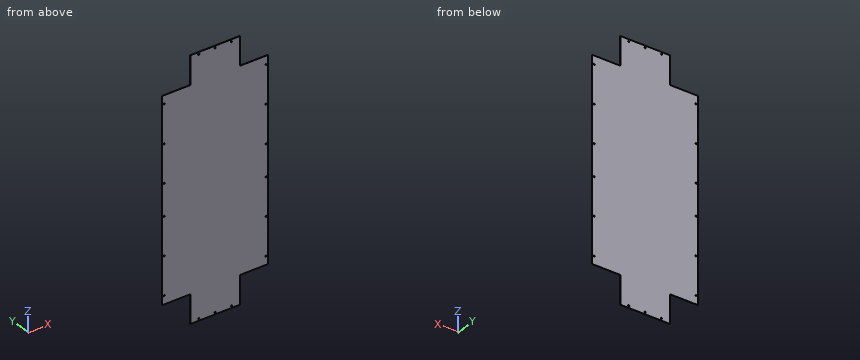
```python
from build123d import *

# Parameters (mm, degrees)
BASE_FLANGE1_DEPTH = 1
SKETCH6_R          = 3
CUT_EXTRUDE1_DEPTH = 10


# Sheet-metal steps are written as plain solids
with BuildPart() as part:
    # Sketch1 → Base-Flange1 (new body)
    with BuildSketch(Plane(origin=(0, 0, 0), x_dir=(1, 0, 0), z_dir=(0, 1, 0))):
        Polygon((135, 0), (371, 0), (371, 135), (506, 135), (506, 1085), (371, 1085), (371, 1220), (135, 1220), (135, 1085), (0, 1085), (0, 135), (135, 135), align=None)
    extrude(amount=-BASE_FLANGE1_DEPTH)

    # Sketch6 → Cut-Extrude1 (cut)
    with BuildSketch(Plane(origin=(0, 0, 0), x_dir=(1, 0, 0), z_dir=(0, 1, 0))):
        with Locations(Location((496, 1045, 0), (0, 0, 270))):
            Circle(SKETCH6_R)
        with Locations(Location((496, 865, 0), (0, 0, 270))):
            Circle(SKETCH6_R)
        with Locations(Location((496, 685, 0), (0, 0, 270))):
            Circle(SKETCH6_R)
        with Locations(Location((331, 1210, 0), (0, 0, 270))):
            Circle(SKETCH6_R)
        with Locations(Location((175, 1210, 0), (0, 0, 270))):
            Circle(SKETCH6_R)
        with Locations(Location((10, 685, 0), (0, 0, 270))):
            Circle(SKETCH6_R)
        with Locations(Location((10, 865, 0), (0, 0, 270))):
            Circle(SKETCH6_R)
        with Locations(Location((10, 1045, 0), (0, 0, 270))):
            Circle(SKETCH6_R)
        with Locations(Location((253, 1209.997298013, 0), (0, 0, 270))):
            Circle(SKETCH6_R)
        with Locations(Location((253, 10.002701987, 0), (0, 0, 270))):
            Circle(SKETCH6_R)
        with Locations(Location((10, 175, 0), (0, 0, 270))):
            Circle(SKETCH6_R)
        with Locations(Location((10, 355, 0), (0, 0, 270))):
            Circle(SKETCH6_R)
        with Locations(Location((10, 535, 0), (0, 0, 270))):
            Circle(SKETCH6_R)
        with Locations(Location((175, 10, 0), (0, 0, 270))):
            Circle(SKETCH6_R)
        with Locations(Location((331, 10, 0), (0, 0, 270))):
            Circle(SKETCH6_R)
        with Locations(Location((496, 535, 0), (0, 0, 270))):
            Circle(SKETCH6_R)
        with Locations(Location((496, 355, 0), (0, 0, 270))):
            Circle(SKETCH6_R)
        with Locations(Location((496, 175, 0), (0, 0, 270))):
            Circle(SKETCH6_R)
    extrude(amount=-CUT_EXTRUDE1_DEPTH, mode=Mode.SUBTRACT)


solid = part.part
```
Read the model definition and answer for the solid it produces. Units are mm, in the model's axes. Round coordinates to 2 decimals unless told otherwise and drop trailing zeros. Write each loop counter-clockwise with the first axis right and the second up, starting at its lowest first coordinate (ties: lowest second). Pieces come first, ordered by that corner, then holes. Notation, with made-up numbers: (88.25, 18) -> (121.25, 18) arc R33 ccw to (121.25, 53) -> close; hole circle Ø3 at (23.25, -32). An arc over 180 degrees is marked (long way). Answer in a Markdown table with one row per item. Add a question column.
1) Consider line 1 (X direction, y = -0.7, z = -10); line 2 (Z direction, x = 253, y = -0.3); line 3 (X direction, y = -0.5, z = -1099). Determine where each line is inside the solid, lowest interval first.
2) Find section B-B, the plane x = 107.5. Determine the outline of the cut face in (y, z).
3) Given P1, Ø5.5, axis at x = 496, z = -865, coming from the +Y side; P2, Ø1, axis at x = 121, z = -505.5, coming from the +Y side; P3, Ø0.5, axis at x = 92, y = -0.5, coming from the -Z side, each flat-ended and moving along its own axis, determine where each tip first touches the part or whether it passes through.
4) Find section A-A, the plane y = -0.5. State how many separate pieces and enclosed holes the cut face has, and give its area (3 significant figures).
Findings below:
| question | item | result |
|---|---|---|
| 1 | line 1 | 135 to 172, 178 to 250, 256 to 328, 334 to 371 |
| 1 | line 2 | -1220 to -1213, -1207 to -13, -7 to 0 |
| 1 | line 3 | 135 to 371 |
| 2 | outline | (-1, -1085) -> (0, -1085) -> (0, -135) -> (-1, -135) -> close |
| 3 | P1 | through |
| 3 | P2 | y = 0 |
| 3 | P3 | z = -1085 |
| 4 | separate pieces | 1 |
| 4 | enclosed holes | 18 |
| 4 | area | 544,000 mm² |
